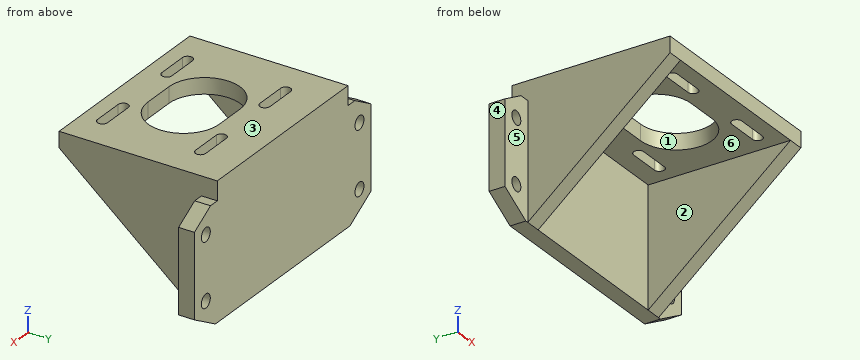
Autodesk Inventor part; units mm, degrees
ref_plane "XZ Plane" through (0, 0, 0) normal (0, 1, 0) x (-1, 0, 0)
ref_plane "XY Plane" through (0, 0, 0) normal (0, 0, 1) x (1, 0, 0)
ref_plane "Work Plane1" through (-118.9196, 128.4425, 80.2184) normal (0, -1, 0) x (0, 0, -1)
sketch "Sketch1" plane through (-118.9196, 128.4425, 80.2184) normal (0, -1, 0) x (0, 0, -1)
  line L0 (-4.2, -124) -> (-4.2, 744) construction
  line L1 (15.8, -124) -> (15.8, 744) construction
  line L2 (25.8, 100) -> (25.8, 520) construction
  line L3 (-12.85, -73.15) -> (24.8, -73.15)
  line L4 (24.8, -73.15) -> (24.8, 11.85)
  line L5 (24.8, 11.85) -> (-12.85, 11.85)
  line L6 (-12.85, 11.85) -> (-12.85, -73.15)
  line L7 (25.8, -30.65) -> (5.6685, -30.65) construction
  circle A0 centre (15.8, -67.65) radius 5.5 construction
  circle A1 centre (15.8, 6.35) radius 5.5 construction
  line L8 (5.8, -58.8473) -> (5.8, 42.3952) construction
  circle A2 centre (-4.2, -67.65) radius 5.5 construction
  circle A3 centre (-4.2, 6.35) radius 5.5 construction
  point P0 (80.2184, 118.9196)
  point P1 (18.9754, -73.15)
  point P2 (24.8, -26.5615)
  dimension "d0" = 1
  dimension "d1" = 38.65
  dimension "d3" = 11
  dimension "d4" = 63
  dimension "d7" = 0
  dimension "d9" = 10
  dimension "d10" = 10
extrude "Extrusion1" add sketch "Sketch1" along normal blind 5
ref_plane "Work Plane2" through (-149.5696, 123.4425, 93.0684) normal (1, 0, 0) x (0, 1, 0)
sketch "Sketch4" plane through (-192.0696, 128.4425, 93.0684) normal (0, 0, 1) x (1, 0, 0)
  line L0 (85, 0) -> (0, 0) construction
  line L1 (0, 0) -> (0, -5) construction
  line L2 (85, -5) -> (0, -5) construction
  line L3 (85, 0) -> (85, -5) construction
  line L4 (0, 0) -> (85, 0) construction
  line L5 (42.5, 0) -> (42.5, -58.6666) construction
  line L6 (11, 0) -> (74, 0)
  line L7 (74, 0) -> (74, -50)
  line L8 (74, -50) -> (11, -50)
  line L9 (11, -50) -> (11, 0)
  line L10 (27, -43.5) -> (58, -43.5) construction
  line L11 (58, -43.5) -> (58, -12.5) construction
  line L12 (58, -12.5) -> (27, -12.5) construction
  line L13 (27, -12.5) -> (27, -43.5) construction
  line L14 (27, -43.5) -> (58, -12.5) construction
  line L15 (58, -43.5) -> (27, -12.5) construction
  line L16 (32, -12.5) -> (22, -12.5) construction
  line L17 (32, -10.9) -> (22, -10.9)
  line L18 (22, -14.1) -> (32, -14.1)
  arc A0 (32, -14.1) -> (32, -10.9) centre (32, -12.5) ccw
  arc A1 (22, -10.9) -> (22, -14.1) centre (22, -12.5) ccw
  line L19 (53, -12.5) -> (63, -12.5) construction
  line L20 (53, -14.1) -> (63, -14.1)
  line L21 (63, -10.9) -> (53, -10.9)
  arc A2 (53, -10.9) -> (53, -14.1) centre (53, -12.5) ccw
  arc A3 (63, -14.1) -> (63, -10.9) centre (63, -12.5) ccw
  line L22 (32, -43.5) -> (22, -43.5) construction
  line L23 (32, -45.1) -> (22, -45.1)
  line L24 (22, -41.9) -> (32, -41.9)
  arc A4 (32, -45.1) -> (32, -41.9) centre (32, -43.5) ccw
  arc A5 (22, -41.9) -> (22, -45.1) centre (22, -43.5) ccw
  line L25 (53, -43.5) -> (63, -43.5) construction
  line L26 (53, -45.1) -> (63, -45.1)
  line L27 (63, -41.9) -> (53, -41.9)
  arc A6 (53, -41.9) -> (53, -45.1) centre (53, -43.5) ccw
  arc A7 (63, -45.1) -> (63, -41.9) centre (63, -43.5) ccw
  line L28 (37.5, -28) -> (47.5, -28) construction
  line L29 (37.5, -39.25) -> (47.5, -39.25)
  line L30 (47.5, -16.75) -> (37.5, -16.75)
  arc A8 (37.5, -16.75) -> (37.5, -39.25) centre (37.5, -28) ccw
  arc A9 (47.5, -39.25) -> (47.5, -16.75) centre (47.5, -28) ccw
  point P0 (192.0696, -128.4425)
  point P1 (42.5, -28)
  dimension "d14" = 63
  dimension "d15" = 45
  dimension "d16" = 31
  dimension "d17" = 31
  dimension "d18" = 3.2
  dimension "d19" = 10
  dimension "d21" = 10
  dimension "d22" = 1.6
  dimension "d23" = 10
  dimension "d24" = 10
  dimension "d25" = 1.6
  dimension "d26" = 1.6
  dimension "d27" = 22.5
  dimension "d28" = 10
extrude "Extrusion2" add sketch "Sketch4" along normal blind 5
sketch "Sketch5" plane through (-181.0696, 78.4425, 93.0684) normal (-1, 0, 0) x (0, 0, 1)
  line L0 (0, 45) -> (0, 0)
  line L1 (0, 45) -> (-37.65, 45)
  line L2 (-37.65, 50) -> (-37.65, 45)
  line L3 (0, 0) -> (0, 45)
  line L4 (-37.65, 45) -> (0, 0)
  point P0 (-93.0684, -78.4425)
extrude "Extrusion3" add sketch "Sketch5" against normal blind 5
sketch "Sketch6" plane through (-118.0696, 78.4425, 93.0684) normal (1, 0, 0) x (0, 0, -1)
  line L0 (0, 0) -> (37.65, 45)
  line L1 (0, 45) -> (37.65, 45)
  line L2 (0, 0) -> (0, 45)
  point P0 (93.0684, -78.4425)
extrude "Extrusion4" add sketch "Sketch6" against normal blind 5
sketch "Sketch7" plane through (-118.9196, 123.4425, 80.2184) normal (0, -1, 0) x (1, 0, 0)
  circle A0 centre (-67.65, -15.8) radius 5.5 construction
  circle A1 centre (-67.65, 4.2) radius 5.5 construction
  circle A2 centre (6.35, 4.2) radius 5.5 construction
  circle A3 centre (6.35, -15.8) radius 5.5 construction
  point P0 (118.9196, -80.2184)
hole "Hole1" at (-186.5696, 123.4425, 84.4184) at (-186.5696, 123.4425, 64.4184) at (-112.5696, 123.4425, 64.4184) at (-112.5696, 123.4425, 84.4184) direction (0, 1, 0) diameter 4.3 end through all
sketch "Sketch8" plane through (-118.9196, 123.4425, 80.2184) normal (0, -1, 0) x (1, 0, 0)
  circle A0 centre (-67.65, 4.2) radius 2.15
  circle A1 centre (-67.65, -15.8) radius 2.15
  line L0 (-62.15, -24.8) -> (-62.15, 12.85)
  line L1 (-62.15, 12.85) -> (-73.15, 12.85)
  line L2 (-73.15, 12.85) -> (-73.15, -24.8)
  line L3 (-73.15, -24.8) -> (-62.15, -24.8)
  circle A2 centre (6.35, -15.8) radius 2.15
  circle A3 centre (6.35, 4.2) radius 2.15
  line L4 (0.85, 12.85) -> (0.85, -24.8)
  line L5 (0.85, -24.8) -> (11.85, -24.8)
  line L6 (11.85, -24.8) -> (11.85, 12.85)
  line L7 (11.85, 12.85) -> (0.85, 12.85)
  line L8 (-73.15, 7.3754) -> (-65.3998, 11.85)
  line L9 (-73.15, -18.9754) -> (-62.15, -25.3263)
  line L10 (11.85, 7.3754) -> (4.0998, 11.85)
  line L11 (11.85, -18.9754) -> (0.85, -25.3263)
  line L12 (-65.3998, 11.85) -> (-62.15, 11.85)
  line L13 (4.0998, 11.85) -> (0.85, 11.85)
  point P0 (118.9196, -80.2184)
  point P1 (37.3678, 12.85)
  point P2 (-28.6678, 12.85)
  point P3 (1.7615, -24.8)
  point P4 (-63.0615, -24.8)
  point P5 (37.3678, 12.85)
  dimension "d42" = 60
  dimension "d43" = 5.5
  dimension "d44" = 60
  dimension "d45" = 5.5
  dimension "d46" = 60
  dimension "d47" = 5.5
  dimension "d48" = 60
  dimension "d49" = 5.5
  dimension "d53" = 7.65
  dimension "d54" = 7.65
extrude "Extrusion5" cut sketch "Sketch8" against normal blind 5 contours L12 L8 L2 L1 L0 | L3 L2 L9 | L7 L6 L10 L13 L4 | L11 L6 L5
equation "\"d1\" = MOTOR_HEIGHT"
equation "\"d9\" = d10"
equation "\"d19\" = SLOT_PLAY"
equation "\"d21\" = d19"
equation "\"d22\" = 0.5 * d18"
equation "\"d23\" = d19"
equation "\"d24\" = d19"
equation "\"d25\" = d22"
equation "\"d26\" = d22"
equation "\"d28\" = SLOT_PLAY"
equation "\"d44\" = d42"
equation "\"d45\" = d43"
equation "\"d47\" = d43"
equation "\"d49\" = d45"
equation "\"d54\" = d53"
equation "\"MOTOR_HEIGHT\" = 38.65"
equation "\"SLOT_PLAY\" = 10"
properties part number "MotorBracketV2"
The listing builds one solid part. Answer for the finished solid, in the listing's coordinates (mm). Face numbers are marked on the shaded views. A direction names the side the tool comes from. Coordinates: 2 decimals unless noted, no trailing zeros. Order: outer loops, then holes, each group sorted by start corner. A loop starts at its lowest first (then second) coordinate and runs counter-clockwise, first axis right, second up.
Q1. A cutting plane is placed at D-D, the plane z = 91. Write down the section's boundary in (x, y), and give its area (3 significant figures).
Q2. Consider line 1 (Y direction, x = -169.5, z = 95.5); line 2 (X direction, y = 117, z = 86); line 3 (Y direction, x = -132, z = 60). Determine where each line is inside the solid, lowest interval first.
Q3. For a pull along X with two mould halves and no side action, classify the marked faces 4, 5 and 6 as pulls with the +X half, pulls with the -X half, needs draft (parallel to the pull), parting line crosses it, or undercut.
Q4. Which of the six approach directions +Z, -Z, +X, -X, +Y, -Y give full straight-line access (tool end or side, diameter ignored) to the marked faces 1, 2 and 3?
Q5. A cutting plane is placed at C-C, the plane x = -111.5. Write down the section's boundary in (y, z).
Q6. A cutting plane is placed at A-A, the plane y = 110.5. Write down the section's boundary in (x, z), and give its area (3 significant figures).
Q7. Given P1, Ø4, axis at x = -181, z = 85.5, coming from the -Y side; P2, Ø6, axis at y = 114.5, z = 62.5, coming from the +X side; P3, Ø5, axis at x = -122.5, y = 100.5, coming from the -Z side, each flat-ended and moving along its own axis, determine where each tip first touches the part or whether it passes through.
Q8. A cutting plane is placed at B-B, the plane x = -155.5. Write down the section's boundary in (y, z).
Answers follow:
1. outline: (-186.17, 123.44) - (-181.07, 123.44) - (-181.07, 80.91) - (-176.07, 80.91) - (-176.07, 123.44) - (-123.07, 123.44) - (-123.07, 80.91) - (-118.07, 80.91) - (-118.07, 123.44) - (-112.97, 123.44) - (-112.97, 128.44) - (-186.17, 128.44) - close
1. area: 791 mm2
2. line 1: y = 78.44 to 83.34, 86.54 to 114.34, 117.54 to 128.44
2. line 2: x = -181.07 to -176.07, -123.07 to -118.07
2. line 3: y = 123.44 to 128.44
3. face 4: pulls with the -X half
3. face 5: needs draft
3. face 6: undercut
4. face 1: +Z, -Z
4. face 2: -Z, -Y
4. face 3: +Z, +X, -X, +Y, -Y
5. outline: (123.44, 58.69) - (128.44, 58.69) - (128.44, 62.55) - (123.44, 62.55) - close; (123.44, 66.28) - (128.44, 66.28) - (128.44, 82.55) - (123.44, 82.55) - close; (123.44, 86.28) - (128.44, 86.28) - (128.44, 90.15) - (123.44, 90.15) - close
6. outline: (-181.07, 66.25) - (-176.07, 66.25) - (-176.07, 93.07) - (-159.61, 93.07) - (-159.61, 98.07) - (-181.07, 98.07) - close; (-139.53, 93.07) - (-123.07, 93.07) - (-123.07, 66.25) - (-118.07, 66.25) - (-118.07, 98.07) - (-139.53, 98.07) - close
6. area: 483 mm2
7. P1: stops at y = 85.1
7. P2: stops at x = -118.07
7. P3: stops at z = 72.52
8. outline: (78.44, 93.07) - (89.23, 93.07) - (89.23, 98.07) - (78.44, 98.07) - close; (111.65, 93.07) - (123.44, 93.07) - (123.44, 55.42) - (128.44, 55.42) - (128.44, 98.07) - (111.65, 98.07) - close
